Geometry: final body of the model. Coordinates: model frame, mm. Round coordinates to 2 decimals unless told otherwise and drop trailing zeros. Loops run counter-clockwise (first coordinate to the right, second up) from the corner with the lowest first, then second, coordinate; pieces in that order, holes last. Notation, with made-up numbers: (10, 32.5) - (15, 32.5) arc R14 cw to (15, 41.5) - close; hole circle Ø10 at (31, -19). An arc over 180 degrees is marked (long way). Answer in a Markdown table with one row per item. Add a question column.
from build123d import *

# Parameters (mm, degrees)
SKETCH1_R           = 40
SKETCH1_R_2         = 20
BOSS_EXTRUDE1_DEPTH = 30
FILLET1_R           = 20


with BuildPart() as part:
    # Sketch1 → Boss-Extrude1 (new body)
    with BuildSketch(Plane(origin=(0, 0, 0), x_dir=(0, 0, -1), z_dir=(1, 0, 0))):
        with BuildLine():
            Line((548.127274586, -214.041985845), (39.098756603, 31.16548142))
            ThreePointArc((39.098756603, 31.16548142), (0, 50), (-39.098756603, 31.16548142))
            Line((-39.098756603, 31.16548142), (-548.127274586, -214.041985845))
            ThreePointArc((-548.127274586, -214.041985845), (-575.897089096, -255.392642304), (-527.11356629, -265.452825709))
            Line((-527.11356629, -265.452825709), (0, -50))
            Line((0, -50), (527.11356629, -265.452825709))
            ThreePointArc((527.11356629, -265.452825709), (575.897089096, -255.392642304), (548.127274586, -214.041985845))
        make_face()
        Circle(SKETCH1_R, mode=Mode.SUBTRACT)
        with Locations((-548.127274586, -244.041985845)):
            Circle(SKETCH1_R_2, mode=Mode.SUBTRACT)
        with Locations((548.127274586, -244.041985845)):
            Circle(SKETCH1_R_2, mode=Mode.SUBTRACT)
    extrude(amount=BOSS_EXTRUDE1_DEPTH)

    # Fillet1
    fillet1_edges = [part.edges().sort_by_distance(p)[0] for p in [
        (15, -265.452825709, -527.11356629),
        (15, -214.041985845, -548.127274586),
        (15, 31.16548142, -39.098756603),
        (15, -214.041985845, 548.127274586),
        (15, 31.16548142, 39.098756603),
        (15, -50, 0),
        (15, -265.452825709, 527.11356629),
    ]]
    fillet(fillet1_edges, radius=FILLET1_R)


solid = part.part
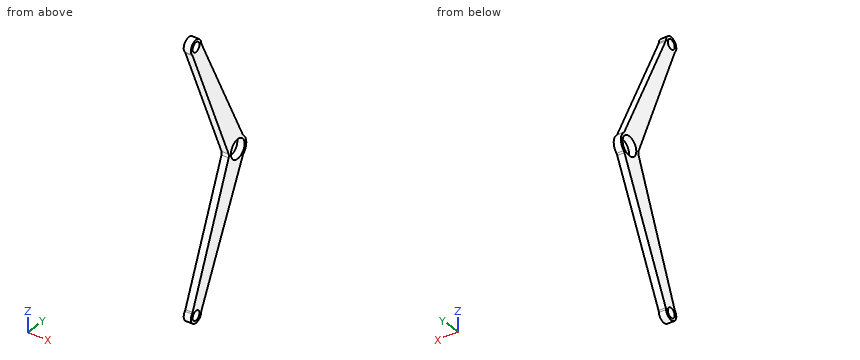
1) Section D-D, the plane z = 376.5. Return the cut outline in (x, y), and give its area (3 significant figures).
2) Section A-A, the plane y = -89.5. Return the cut outline in (x, z), and give its area (3 significant figures).
3) Section B-B, the plane x = 24. Return the cut outline in (y, z).
4) Material intervals for line 1 along Z through (x, y) = (13.5, -231); line 2 along Y through (x, z) = (20, -13); line 3 along Z through (x, y) = (4.5, -240.5), sorted ascending. Write a range as from..to.
5) Section C-C, the plane y = 11. Return the cut outline in (x, z), and give its area (3 significant figures).
6) Contact query for flat-ended pins moving along their axis: pin 1 Ø5 at (x, y) = (22, 8) entering from +Z; pin 2 Ø4 at (x, y) = (14, -180) entering from +Z; pin 3 Ø12 at (x, z) = (17.5, 278.5) entering from +Y. Output: stop coordinate, or through.
Evaluation:
| question | item | result |
|---|---|---|
| 1 | outline | (0, -203.89) - (30, -203.89) - (30, -131.37) - (0, -131.37) - close |
| 1 | area | 2,180 mm² |
| 2 | outline | (0, -289.59) - (30, -289.59) - (30, -96.64) - (0, -96.64) - close; (0, 96.64) - (30, 96.64) - (30, 289.59) - (0, 289.59) - close |
| 2 | area | 11,600 mm² |
| 3 | outline | (-267.22, -529.08) arc R30 ccw (long way) to (-214.2, -551.19) arc R20 cw to (-212.32, -544.56) - (29.36, -42.85) arc R20 cw to (33.84, -36.81) arc R50 ccw to (33.84, 36.81) arc R20 cw to (29.36, 42.85) - (-212.32, 544.56) arc R20 cw to (-214.2, 551.19) arc R30 ccw (long way) to (-267.22, 529.08) arc R20 cw to (-264.16, 523.95) - (-53.09, 7.57) arc R20 cw to (-53.09, -7.57) - (-264.16, -523.95) arc R20 cw to start; hole circle Ø40 at (-244.04, -548.13); hole circle Ø40 at (-244.04, 548.13); hole circle Ø80 at (0, 0) |
| 4 | line 1 | z = -575.14..-563.29, -532.96..-442.82, 442.82..532.96, 563.29..575.14 |
| 4 | line 2 | y = -55.31..-37.83, 37.83..48.28 |
| 4 | line 3 | z = -577.92..-567.81, -528.44..-466.07, 466.07..528.44, 567.81..577.92 |
| 5 | outline | (0, -80.96) - (30, -80.96) - (30, -38.46) - (0, -38.46) - close; (0, 38.46) - (30, 38.46) - (30, 80.96) - (0, 80.96) - close |
| 5 | area | 2,550 mm² |
| 6 | pin 1 | stops at z = 92.38 |
| 6 | pin 2 | stops at z = 481.61 |
| 6 | pin 3 | stops at y = -81.27 |
